Verification items for the finished model (mm, model axes). A direction names the side the tool comes from. Coordinates: 2 decimals unless noted, no trailing zeros. Order: outer loops, then holes, each group sorted by start corner. A loop starts at its lowest first (then second) coordinate and runs counter-clockwise, first axis right, second up. Notation, with made-up numbers: M 80.25,2 L 96.25,2 A32 cw 96.25,36 Z; hole C 89,26.5 d5. An arc over 180 degrees is marked long. Return JSON: item names as keys, results as strings. Group by question number.
1. Mould release check, pull along X, two halves, no side actions. Record for faces 1 (the flat face through (0, -47, -6.339)), 2 (the flat face through (-13.041, -47, 0)), 3 (the flat face through (0, 8, 0)): +X half, -X half, draft (parallel to the pull), parting line (faces both ways), or undercut.
2. Gauge pin test, flat ends, axial feed: pin 1 (16.5 mm diameter, centred on x = 1.5, y = -51, fed in from -Z); pin 2 (14 mm diameter, centred on y = -44.5, z = 3, fed in from -X); pin 3 (4 mm diameter, centred on y = -47.5, z = 2.5, fed in from +X). Record the tip position at first contact, or that the pin passes through.
3. Set-up check for faces 4 (the cylindrical face through (5.554, -19.72, 13.394)), 5 (the flat face through (0, -40, -10)), 6 (the flat face through (-14, -40, 0)), 7 (the flat face through (0, -47, 6.339)), 8 (the flat face through (13.041, -47, 0)): record each of +Z, -Z, +X, -X, +Y, -Y from which the full face is reachable in a straight line by a thin tool's end or side.
4. Section check B-B, the plane y = -45. Record the cut outline in (x, z), plus the area to 3 significant figures.
5. Material ranges on line 1 along Z through (x, y) = (-4, -48); line 2 along Y through (x, z) = (-11.5, -1); line 3 along Z through (x, y) = (-4.5, -4.5), recorded low to high.
6. Section check A-A, the plane y = -34. Record the cut outline in (x, z).
```python
from build123d import *

# Parameters (mm, degrees)
SKETCH1_R           = 17.5
BOSS_EXTRUDE1_DEPTH = 5
FILLET1_R           = 5
SKETCH2_R           = 12.5
BOSS_EXTRUDE2_DEPTH = 4
FILLET2_R           = 1
SKETCH3_R           = 11.5
CUT_EXTRUDE1_DEPTH  = 1
FILLET5_R           = 57
SKETCH5_R           = 14.5
BOSS_EXTRUDE3_DEPTH = 40
SKETCH6_W           = 26.081932022
SKETCH6_H           = 12.67804488
BOSS_EXTRUDE4_DEPTH = 15


# Some blends are built 0.0001 mm under size
with BuildPart() as part:
    # Sketch1 → Boss-Extrude1 (new body)
    with BuildSketch(Plane(origin=(0, 0, 0), x_dir=(1, 0, 0), z_dir=(0, 1, 0))):
        with Locations(Location((0, 0, 0), (0, 0, 270))):
            Circle(SKETCH1_R)
    extrude(amount=BOSS_EXTRUDE1_DEPTH)

    # Fillet1
    fillet1_edges = [part.edges().sort_by_distance(p)[0] for p in [
        (0, 5, -17.5),
    ]]
    fillet(fillet1_edges, radius=FILLET1_R - 0.0001)  # a hair under: the kernel refuses the full size

    # Sketch2 → Boss-Extrude2 (add)
    with BuildSketch(Plane(origin=(0, 5, 0), x_dir=(1, 0, 0), z_dir=(0, 1, 0))):
        with Locations(Location((0, 0, 0), (0, 0, 270))):
            Circle(SKETCH2_R)
    extrude(amount=BOSS_EXTRUDE2_DEPTH)

    # Fillet2
    fillet2_edges = [part.edges().sort_by_distance(p)[0] for p in [
        (0, 9, -12.5),
    ]]
    fillet(fillet2_edges, radius=FILLET2_R)

    # Sketch3 → Cut-Extrude1 (cut)
    with BuildSketch(Plane(origin=(0, 9, 0), x_dir=(1, 0, 0), z_dir=(0, 1, 0))):
        with Locations(Location((0, 0, 0), (0, 0, 270))):
            Circle(SKETCH3_R)
    extrude(amount=-CUT_EXTRUDE1_DEPTH, mode=Mode.SUBTRACT)

    # Fillet5
    # the kernel refuses this fillet: 57 mm, written as the material it adds along each edge
    with BuildSketch(Plane(origin=(0, 8, 0), x_dir=(0, 0, 1), z_dir=(-1, 0, 0))) as fillet5_piece_1:
        with BuildLine():
            CenterArc((0.869854187, 57), FILLET5_R, 270, 10.748235858)
            Line((0.869854187, 0), (11.5, 0))
            Line((11.5, 0), (11.5, 1))
        make_face()
    revolve(axis=Axis((0, 8, 0), (0, 1, 0)))

    # Sketch5 → Boss-Extrude3 (add)
    with BuildSketch(Plane.XZ):
        with Locations(Location((0, 0, 0), (0, 0, 90))):
            Circle(SKETCH5_R)
    extrude(amount=BOSS_EXTRUDE3_DEPTH)

    # Sketch6 → Boss-Extrude4 (add)
    with BuildSketch(Plane.XZ.offset(40)):
        Rectangle(SKETCH6_W, SKETCH6_H)
    extrude(amount=BOSS_EXTRUDE4_DEPTH)


solid = part.part
```
Answers follow:
{
 "1": {"face 1": "draft", "face 2": "-X half", "face 3": "undercut"},
 "2": {"pin 1": "z = -6.34", "pin 2": "x = -14.5", "pin 3": "x = 13.04"},
 "3": {"face 4": "-Y", "face 5": "-Z, +X, -X, -Y", "face 6": "+Z, -Z, -X, -Y", "face 7": "+Z, +X, -X, -Y", "face 8": "+Z, -Z, +X, -Y"},
 "4": {"outline": "M -13.04,-6.34 L 13.04,-6.34 L 13.04,6.34 L -13.04,6.34 Z", "area": "331 mm^2"},
 "5": {"line 1": "-6.34 to 6.34", "line 2": "-55 to 9", "line 3": "-13.78 to 13.78"},
 "6": {"outline": "C 0,0 d29"}
}
